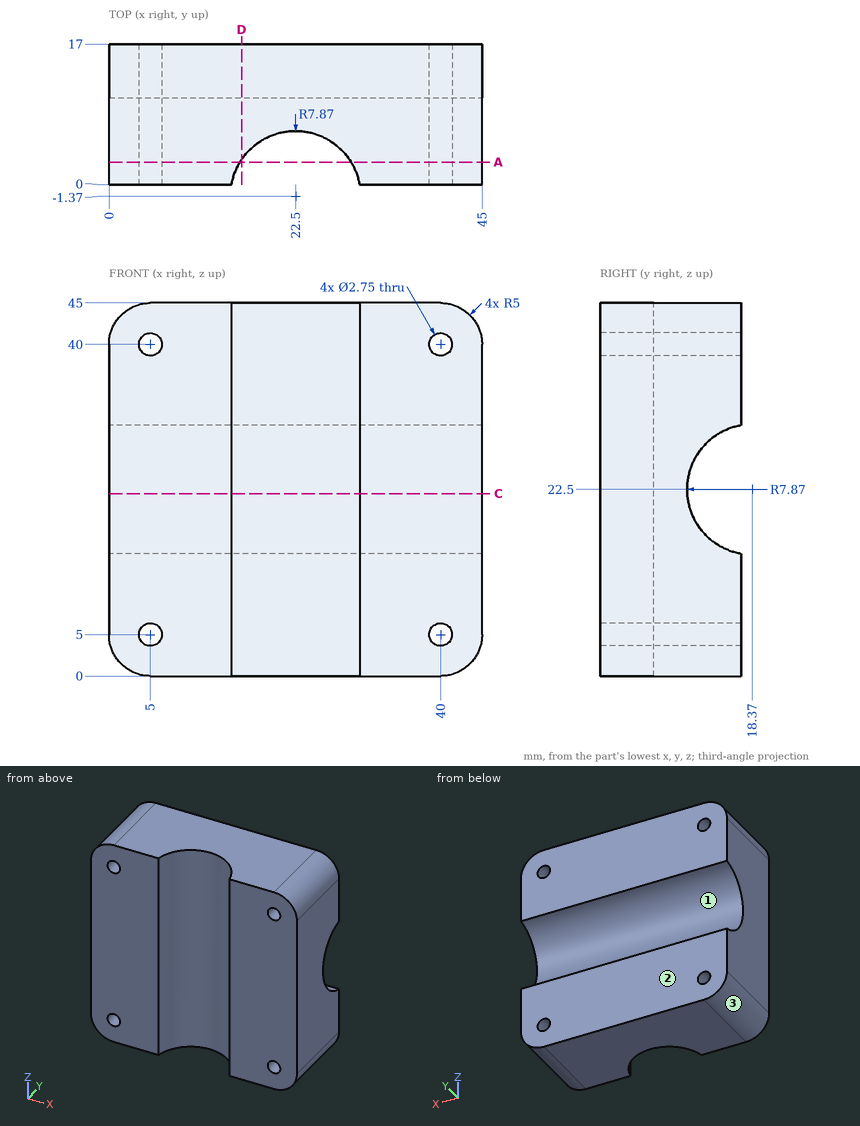
Print and shaded views of the part. All mm, measured from the part's lowest x, y and z. Round coordinates to 2 decimals unless told otherwise and drop trailing zeros. Write each loop counter-clockwise with the first axis right and the second up, starting at its lowest first coordinate (ties: lowest second). Pieces come first, ordered by that corner, then holes. Notation, with made-up numbers: (66.5, 23.5) -> (74.5, 23.5) arc R13 cw to (74.5, 38.5) -> close; hole circle Ø4 at (3, 74). An arc over 180 degrees is marked (long way). Return JSON: item names as keys, results as strings. Group by question number.
Q1. Saw through at D-D on x = 16. Write the cut outline in (y, z), plus the area to 3 significant figures.
Q2. Mould opens along Z. For the marked faces 1, 2 and 3 say: pulls with the +Z half, pulls with the -Z half, needs draft (parallel to the pull), parting line crosses it, or undercut.
Q3. Saw through at C-C on z = 22. Write the cut outline in (x, y), plus the area to 3 significant figures.
Q4. Saw through at A-A on y = 2.75. State how many separate pieces and enclosed holes the cut face has, plus the area to 3 significant figures.
Q5. Probe L1, parallel to Z at x = 40, y = 5 (3 decimals); L2, parallel to Z at x = 40, y = 13 (1 decimal); L3, parallel to Z at x = 41, y = 16 (1 decimal). List the from-to ranges inside material, lowest first. Write a range as [from, to].
Q6. Pin check, flat tips, straight feed: pin 1 (2 mm diameter, centred on y = 7.5, z = 32, fed in from -X); pin 2 (2 mm diameter, centred on x = 5, z = 40, fed in from -Y). Stop position of each tip, or through.
Answer:
{
 "1": {"outline": "(3.07, 0) -> (17, 0) -> (17, 14.75) arc R7.87 cw to (17, 30.25) -> (17, 45) -> (3.07, 45) -> close", "area": "551 mm2"},
 "2": {"face 1": "undercut", "face 2": "needs draft", "face 3": "pulls with the -Z half"},
 "3": {"outline": "(0, 0) -> (14.75, 0) arc R7.87 cw to (30.25, 0) -> (45, 0) -> (45, 10.52) -> (0, 10.52) -> close", "area": "397 mm2"},
 "4": {"separate pieces": "2", "enclosed holes": "4", "area": "1,380 mm2"},
 "5": {"L1": "[0, 3.625], [6.375, 38.625], [41.375, 45]", "L2": "[0, 3.6], [6.4, 16.7], [28.3, 38.6], [41.4, 45]", "L3": "[0.1, 4.1], [5.9, 15], [30, 39.1], [40.9, 44.9]"},
 "6": {"pin 1": "x = 0", "pin 2": "through"}
}
